For this review, take the finished solid that the model builds, in its own axes (mm). A direction names the side the tool comes from. Coordinates: 2 decimals unless noted, no trailing zeros. Loops run counter-clockwise (first coordinate to the right, second up) from the corner with the lowest first, then second, coordinate; pieces in that order, holes last. Notation, with made-up numbers: (80.25, 4.5) - (106.25, 4.5) arc R18 cw to (106.25, 23.5) - close; hole circle Ø8 at (-12.75, -3.75). An arc over 180 degrees is marked (long way). One line per item, written item: value. Start each with the question number.
1. Take a section at A-A, the plane y = 59. State the section outline as (x, z) points, and give its area (3 significant figures).
2. For faces 5 (the face through (-1.7, -93.7, -6)), 6 (the face through (61, -16, -7)), 7 (the face through (62.01, 43.55, -6.54)), list the 3-axis set-ups (+Z, -Z, +X, -X, +Y, -Y) from which the entire face can be reached by the end or side of a thin tool; tool diameter is ignored.
3. Take a section at B-B, the plane x = -34. State the section outline as (y, z) points, and give its area (3 significant figures).
4. Insertion check: pin 1 (2 mm diameter, centred on x = -0.5, y = -39, fed in from -Z); pin 2 (0.8 mm diameter, centred on x = 62, z = -8.5, fed in from +Y); pin 3 (2.5 mm diameter, centred on y = 41.5, z = -7, fed in from -X). Each pin has a flat end and moves straight along its axis. Give the tip position at first contact, or say it passes through.
5. Take a section at C-C, the plane y = -47. State the section outline as (x, z) points.
6. Take a section at D-D, the plane z = -34.5. State the section outline as (x, y) points.
7. The part is to be moulded in two halves that separate along Y. For faces 1 (the face through (6.51, 110.01, -40.49)), 2 (the face through (-43.8, 56.68, -1.01)), 3 (the face through (-61.574, 85.606, -95.956)), 4 (the face through (-55.34, 92.93, -85.3)), say which applies: released by +Y, released by -Y, zero draft, split by the parting line, or undercut.
8. To check wall thickness, follow line 1 (X direction, y = 109.95, z = -29); line 2 (X direction, y = -95, z = -4.25); line 3 (Z direction, x = -46, y = -0.5). State the ranges of each line that lie inside material, in increasing order. Write a range as from..to.
```python
from build123d import *

# Parameters (mm, degrees)
SM_BASE_FLANGE_1_DEPTH = 111
CUT_EXTRUDE_1_REACH    = 170.348
SKETCH_3_W             = 10
SKETCH_3_H             = 35
EXTRUDE_1_DEPTH        = 4
M4X0_7_1_D             = 3.3
SKETCH_8_R             = 2.75
CUT_EXTRUDE_2_DEPTH    = 129.023435355
M5X0_8_1_AT_2_COUNT    = 2
M5X0_8_1_AT_2_PITCH    = 140
EXTRUDE_2_DEPTH        = 48
SKETCH_12_R            = 19
CUT_EXTRUDE_3_DEPTH    = 2
SKETCH_13_R            = 19
CUT_EXTRUDE_4_DEPTH    = 2
FILLET_1_R             = 5
SKETCH_14_W            = 51.6317
SKETCH_14_H            = 2
EXTRUDE_3_DEPTH        = 40
CUT_EXTRUDE_5_REACH    = 252.621
SKETCH_15_R            = 11.5
FILLET_2_R             = 5


# Sheet-metal steps are written as plain solids
with BuildPart() as part:
    # Sketch 1 → 基体-法兰1 (new, symmetric)
    with BuildSketch(Plane(origin=(0, 0, 0), x_dir=(1, 0, 0), z_dir=(0, 1, 0))):
        with BuildLine():
            Line((-63, 12), (-63, 2.7366))
            ThreePointArc((-63, 2.7366), (-62.198468417, 0.801531583), (-60.2634, 0))
            Line((-60.2634, 0), (60.2634, 0))
            ThreePointArc((60.2634, 0), (62.198468417, 0.801531583), (63, 2.7366))
            Line((63, 2.7366), (63, 12))
            Line((63, 12), (61, 12))
            Line((61, 12), (61, 2.7366))
            ThreePointArc((61, 2.7366), (60.784254855, 2.215745145), (60.2634, 2))
            Line((60.2634, 2), (-60.2634, 2))
            ThreePointArc((-60.2634, 2), (-60.784254855, 2.215745145), (-61, 2.7366))
            Line((-61, 2.7366), (-61, 12))
            Line((-61, 12), (-63, 12))
        make_face()
    extrude(amount=SM_BASE_FLANGE_1_DEPTH, both=True)

    # 草图3 → 切除-拉伸1 (cut, up to next)
    with BuildSketch(Plane(origin=(63, 0, 0), x_dir=(0, 0, -1), z_dir=(1, 0, 0)), mode=Mode.PRIVATE) as cut_extrude_1_sk1:
        with Locations((7, 93.5)):
            Rectangle(SKETCH_3_W, SKETCH_3_H)
    cut_extrude_1_tool1 = extrude(cut_extrude_1_sk1.sketch, amount=-CUT_EXTRUDE_1_REACH, mode=Mode.PRIVATE) & part.part
    add(cut_extrude_1_tool1.solids().sort_by_distance((63, 93.5, -7))[0], mode=Mode.SUBTRACT)

    # 草图4 → 凸台-拉伸1 (add)
    with BuildSketch(Plane(origin=(0, 0, -2), x_dir=(-1, 0, 0), z_dir=(0, 0, -1))):
        Polygon((-14.987954458, 43.07002562), (-17.786672003, 43.777495363), (-19.798717545, 41.707469743), (-19.012045542, 38.92997438), (-16.213327997, 38.222504637), (-14.201282455, 40.292530257), align=None)
        Polygon((5.723956961, 41.955715338), (3.534304719, 43.836873596), (0.810347758, 42.881158258), (0.276043039, 40.044284662), (2.465695281, 38.163126404), (5.189652242, 39.118841742), align=None)
        Polygon((-15.276915043, -92.683901651), (-18.14425753, -92.34971548), (-19.867342487, -94.665813829), (-18.723084957, -97.316098349), (-15.85574247, -97.65028452), (-14.132657513, -95.334186171), align=None)
        Polygon((5.052579277, -92.9701597), (2.268396373, -92.207494053), (0.215817096, -94.237334353), (0.947420723, -97.0298403), (3.731603627, -97.792505947), (5.784182904, -95.762665647), align=None)
    extrude(amount=EXTRUDE_1_DEPTH)

    # M4x0.7 螺纹孔1 (through all)
    with Locations(Plane(origin=(0, 0, -6), x_dir=(-1, 0, 0), z_dir=(0, 0, -1))):
        with Locations((-17, 41), (3, 41), (-17, -95), (3, -95)):
            Hole(M4X0_7_1_D / 2)

    # 草图8 → 切除-拉伸2 (cut, through all)
    with BuildSketch(Plane(origin=(0, 0, -2), x_dir=(-1, 0, 0), z_dir=(0, 0, -1))):
        with Locations((-44.723956961, 59)):
            Circle(SKETCH_8_R)
        with Locations(Location((45.276043039, 59, 0), (0, 0, 180))):
            Circle(SKETCH_8_R)
        with Locations((-44.723956961, -101)):
            Circle(SKETCH_8_R)
        with Locations(Location((45.276043039, -101, 0), (0, 0, 180))):
            Circle(SKETCH_8_R)
    extrude(amount=-CUT_EXTRUDE_2_DEPTH, mode=Mode.SUBTRACT)

    # 草图9 → M5x0.8 螺纹孔1 (revolve, cut)
    with BuildSketch(Plane(origin=(63, -98.5, -7), x_dir=(0, 0, -1), z_dir=(0, 1, 0))):
        Polygon((0, 0), (0, 13.6618073), (2.1, 12.4), (2.1, 0), align=None)
    m5x0_8_1 = revolve(axis=Axis((69.35, -98.5, -7), (-1, 0, 0)), mode=Mode.SUBTRACT)

    # M5x0.8 螺纹孔1 at 2: M5x0.8 螺纹孔1 ×2
    with Locations(*[(0, i * M5X0_8_1_AT_2_PITCH, 0) for i in range(1, M5X0_8_1_AT_2_COUNT)]):
        add(m5x0_8_1, mode=Mode.SUBTRACT)

    # 镜向1: M5x0.8 螺纹孔1 across plane
    add(m5x0_8_1.mirror(Plane(origin=(0, 0, 0), x_dir=(0, 0, 1), z_dir=(1, 0, 0))), mode=Mode.SUBTRACT)

    # 镜向1 copy 1 sketch → 镜向1 copy 1 (revolve, cut)
    with BuildSketch(Plane(origin=(-63, 41.5, -7), x_dir=(0, 0, -1), z_dir=(0, 1, 0))):
        Polygon((0, 0), (0, -13.6618073), (2.1, -12.4), (2.1, 0), align=None)
    revolve(axis=Axis((-69.35, 41.5, -7), (-1, 0, 0)), mode=Mode.SUBTRACT)

    # 草图11 → 凸台-拉伸2 (add)
    with BuildSketch(Plane.ZY.offset(63)):
        Polygon((-2, 111), (-54, 111), (-97.765371804, 85.732050808), (-96.765371804, 84), (-53.464101615, 109), (-2, 109), align=None)
    extrude(amount=-EXTRUDE_2_DEPTH)

    # 草图12 → 切除-拉伸3 (cut)
    with BuildSketch(Plane(origin=(0, 111, 0), x_dir=(1, 0, 0), z_dir=(0, 1, 0))):
        with Locations(Location((-39, 29, 0), (0, 0, 270))):
            Circle(SKETCH_12_R)
    extrude(amount=-CUT_EXTRUDE_3_DEPTH, mode=Mode.SUBTRACT)

    # 草图13 → 切除-拉伸4 (cut)
    with BuildSketch(Plane(origin=(0, 106.632685902, -61.56440991), x_dir=(1, 0, 0), z_dir=(0, 0.8660254037844386, -0.5000000000000001))):
        with Locations(Location((-39, 16.533320997, 0), (0, 0, 270))):
            Circle(SKETCH_13_R)
    extrude(amount=-CUT_EXTRUDE_4_DEPTH, mode=Mode.SUBTRACT)

    # 圆角1
    fillet_1_edges = [part.edges().sort_by_distance(p)[0] for p in [
        (-63, 84.866025404, -97.265371804),
        (-15, 84.866025404, -97.265371804),
    ]]
    fillet(fillet_1_edges, radius=FILLET_1_R)

    # 草图14 → 凸台-拉伸3 (add)
    with BuildSketch(Plane(origin=(-15, 0, 0), x_dir=(0, 0, -1), z_dir=(1, 0, 0))):
        with Locations((28.18415, 110)):
            Rectangle(SKETCH_14_W, SKETCH_14_H)
    extrude(amount=EXTRUDE_3_DEPTH)

    # 草图15 → 切除-拉伸5 (cut, up to next)
    with BuildSketch(Plane(origin=(0, 111, 0), x_dir=(1, 0, 0), z_dir=(0, 1, 0)), mode=Mode.PRIVATE) as cut_extrude_5_sk1:
        with Locations(Location((6, 29, 0), (0, 0, 270))):
            Circle(SKETCH_15_R)
    cut_extrude_5_tool1 = extrude(cut_extrude_5_sk1.sketch, amount=-CUT_EXTRUDE_5_REACH, mode=Mode.PRIVATE) & part.part
    add(cut_extrude_5_tool1.solids().sort_by_distance((6, 111, -29))[0], mode=Mode.SUBTRACT)

    # 圆角2
    fillet_2_edges = [part.edges().sort_by_distance(p)[0] for p in [
        (25, 110, -54),
    ]]
    fillet(fillet_2_edges, radius=FILLET_2_R)


solid = part.part
```
Solutions:
1. outline: (-63, -12) - (-61, -12) - (-61, -2.74) arc R0.74 cw to (-60.26, -2) - (-48.03, -2) - (-48.03, 0) - (-60.26, 0) arc R2.74 ccw to (-63, -2.74) - close; (-42.53, -2) - (41.97, -2) - (41.97, 0) - (-42.53, 0) - close; (47.47, -2) - (60.26, -2) arc R0.74 cw to (61, -2.74) - (61, -12) - (63, -12) - (63, -2.74) arc R2.74 ccw to (60.26, 0) - (47.47, 0) - close
1. area: 267 mm2
2. face 5: -Z, -Y
2. face 6: -Z, +Y, -Y
2. face 7: +X
3. outline: (-111, -2) - (109, -2) - (109, -10.67) - (111, -10.67) - (111, 0) - (-111, 0) - close; (84, -96.77) - (85.73, -97.77) - (89.2, -91.76) - (87.47, -90.76) - close; (105.8, -59.01) - (107.53, -60.01) - (111, -54) - (111, -47.33) - (109, -47.33) - (109, -53.46) - close
3. area: 501 mm2
4. pin 1: z = -2
4. pin 2: y = 76
4. pin 3: x = -5.72
5. outline: (-63, -12) - (-61, -12) - (-61, -2.74) arc R0.74 cw to (-60.26, -2) - (60.26, -2) arc R0.74 cw to (61, -2.74) - (61, -12) - (63, -12) - (63, -2.74) arc R2.74 ccw to (60.26, 0) - (-60.26, 0) arc R2.74 ccw to (-63, -2.74) - close
6. outline: (-63, 109) - (-57.19, 109) - (-57.19, 111) - (-63, 111) - close; (-20.81, 109) - (-4.1, 109) - (-4.1, 111) - (-20.81, 111) - close; (16.1, 109) - (25, 109) - (25, 111) - (16.1, 111) - close
7. face 1: zero draft
7. face 2: undercut
7. face 3: released by -Y
7. face 4: released by +Y
8. line 1: -63..-58, -20..-5.5, 17.5..25
8. line 2: -63..-61, -5.58..-4.65, -1.35..-0.42, 14.28..15.35, 18.65..19.72, 61..63
8. line 3: -2..0
